Here's how the part is built. I have some questions about the finished solid (model axes, mm). A direction names the side the tool comes from. Coordinates: 2 decimals unless noted, no trailing zeros. Write each loop counter-clockwise with the first axis right and the second up, starting at its lowest first coordinate (ties: lowest second). Pieces come first, ordered by that corner, then holes.
```python
from build123d import *

# Parameters (mm, degrees)
F2_W     = 431.8
F2_H     = 15.24
F3_DEPTH = 15.24
F5_DEPTH = 51.827874
F6_DEPTH = 67.423307
F7_DEPTH = 254


with BuildPart() as f3:
    # F2 (on face) → F3 (new body)
    with BuildSketch(Plane(origin=(0, 0, 0), x_dir=(0.970296, 0, 0.241922), z_dir=(0.241922, 0, -0.970296))):
        with Locations((1.670222, 0)):
            Rectangle(F2_W, F2_H)
    extrude(amount=-F3_DEPTH)

    # F4 (on Top) → F5 (cut, through all)
    with BuildSketch(Plane.XY):
        Polygon((0, -174.718463), (-227.059232, 52.340768), (-254, 25.4), (0, -228.6), (254, 25.4), (227.059232, 52.340768), align=None)
    extrude(amount=-F5_DEPTH, mode=Mode.SUBTRACT)

    # F4 (on Top) → F6 (cut, through all)
    with BuildSketch(Plane.XY):
        Polygon((0, -174.718463), (-227.059232, 52.340768), (-254, 25.4), (0, -228.6), (254, 25.4), (227.059232, 52.340768), align=None)
    extrude(amount=F6_DEPTH, mode=Mode.SUBTRACT)

    # F4 (on Top) → F7 (join, symmetric)
    with BuildSketch(Plane.XY):
        Polygon((0, -174.718463), (-227.059232, 52.340768), (-254, 25.4), (0, -228.6), (254, 25.4), (227.059232, 52.340768), align=None)
    extrude(amount=F7_DEPTH, both=True)


solid = f3.part
```
1) I need wall thicknesses on probe 1 along X at (y, z) = (-120, 31.5); probe 2 along X at (y, z) = (-166.5, -118.5); probe 3 along Y at (x, z) = (-211, 36.5). Which ranges of each line are inside material? Lowest first, please.
Values follow:
probe 1: x = -108.6 to -54.72, 54.72 to 108.6
probe 2: x = -62.1 to -8.22, 8.22 to 62.1
probe 3: y = -17.6 to 36.28
2) We'd pull the mould along X, two halves only. Please class faces 6 (the face through (-2, -7.62, 7)), 7 (the face through (-58, -119, -254)), 8 (the face through (125.2, -103.4, 3.6)): pulls with the +X half, pulls with the -X half, needs draft (parallel to the pull), parting line crosses it, or undercut.
Values follow:
face 6: undercut
face 7: needs draft
face 8: pulls with the +X half
3) Will these pins go through, and if not, where does the flat tip stop? pin 1 (10 mm diameter, centred on x = -47, z = 69.5, fed in from -Y); pin 2 (8 mm diameter, centred on x = -194.5, z = -143.5, fed in from -Y); pin 3 (1 mm diameter, centred on x = -159.5, z = -116.5, fed in from -Y).
Values follow:
pin 1: stops at y = -186.6
pin 2: stops at y = -38.1
pin 3: stops at y = -69.6
4) Imagine slicing it at A-A on x = 121.5. Please give me the cut outline in (y, z), then the cut area to 3 significant figures.
Values follow:
outline: (-107.1, -254) - (-53.22, -254) - (-53.22, 254) - (-107.1, 254) - close; (-7.62, 30.29) - (7.62, 30.29) - (7.62, 46) - (-7.62, 46) - close
area: 27,600 mm2
5) Imagine slicing it at D-D on y = -181. Please give me the cut outline in (x, z), then the cut area to 3 significant figures.
Values follow:
outline: (-47.6, -254) - (47.6, -254) - (47.6, 254) - (-47.6, 254) - close
area: 48,400 mm2
6) Imagine slicing it at B-B on y = -96. Please give me the cut outline in (x, z), then the cut area to 3 significant figures.
Values follow:
outline: (-132.6, -254) - (-78.72, -254) - (-78.72, 254) - (-132.6, 254) - close; (78.72, -254) - (132.6, -254) - (132.6, 254) - (78.72, 254) - close
area: 54,700 mm2
7) Imagine slicing it at C-C on z = 2. Please give me the cut outline in (x, y), then the cut area to 3 significant figures.
Values follow:
outline: (-254, 25.4) - (0, -228.6) - (254, 25.4) - (227.06, 52.34) - (0, -174.72) - (-227.06, 52.34) - close; (-54.97, -7.62) - (8.02, -7.62) - (8.02, 7.62) - (-54.97, 7.62) - close
area: 26,900 mm2
8) On a 3-axis mill with a long thin cutter (end or side, diameter ignored), from which of +Z, -Z, +X, -X, +Y, -Y can I reach the whole of each face in a straight line? I mean faces 1 (the face through (-2.553, -0.107, -0.636)), 2 (the face through (-58, -119, 254)), 3 (the face through (-128.8, -99.8, 3.6)), 4 (the face through (-2.55, -0.11, 15.07)), 5 (the face through (-3, 7.62, 7)). Say none if no direction works.
Values follow:
face 1: -Z, +Y
face 2: +Z, +X, -X, +Y, -Y
face 3: +Z, -Z, -X, -Y
face 4: +Z, +Y
face 5: +Z, -Z, +Y
